Part model, mm, in its own coordinate system. A direction names the side the tool comes from. Round coordinates to 2 decimals unless told otherwise and drop trailing zeros. Write each loop counter-clockwise with the first axis right and the second up, starting at its lowest first coordinate (ties: lowest second). Pieces come first, ordered by that corner, then holes. Notation, with made-up numbers: M 73.25,75 L 132.25,75 A34 ccw 132.25,107 Z; hole C 9.5,-40 d10. An arc over 180 degrees is marked long. Answer as a JSON object with one key per item and string values. Group by question number.
1. Two-plate mould, pull along Y, no slides. Class faces 4 (the face through (19, -3.175, 0)), 5 (the face through (34.93, 98.29, 0.14)), 6 (the face through (0.69, 81.82, -3.1)): +Y half, -Y half, draft (parallel to the pull), parting line (faces both ways), or undercut.
2. Drill centre lines: line 1 (Y direction, x = 7.5, z = -1); line 2 (Y direction, x = 16.5, z = 0.25) (3 decimals); line 3 (X direction, y = 22, z = -0.25). Where is each one in solid material? Low to high. Write a range as from..to.
3. Which spindle directions (+Z, -Z, +X, -X, +Y, -Y) get a long thin tool onto all of the face, cutting with end or side? Do faces 1 (the face through (38, 88.9, 0)), 2 (the face through (22.22, 11.77, 0.14)), 3 (the face through (11.521, 42.193, -1.932)). Say none if no direction does.
4. Drop flat-ended pins along their axis: pin 1 (1.9 mm diameter, centred on x = 39, z = 1.5, fed in from -Y); pin 2 (2 mm diameter, centred on y = 101.5, z = -2, fed in from +X); pin 3 (1 mm diameter, centred on x = 23.5, y = 19.5, fed in from +Z). Give the stop position or say it passes through.
5. Band-saw the part on A-A, the plane z = 0. Write the cut outline in (x, y) (3 decimals).
6. Band-saw the part on B-B, the plane y = 75. Write the cut outline in (x, z) (3 decimals), plus the area to 3 significant figures.
Autodesk Inventor part; units mm, degrees
ref_plane "Work Plane1" through (19.05, 0, 0) normal (0, 1, 0) x (-1, 0, 0)
ref_plane "YZ Plane" through (0, 0, 0) normal (1, 0, 0) x (0, 1, 0)
ref_plane "XZ Plane" through (0, 0, 0) normal (0, 1, 0) x (-1, 0, 0)
sketch "Sketch1" plane through (0, 0, 0) normal (0, 0, 1) x (1, 0, 0)
  line L0 (19.05, 0) -> (19.05, 25.4)
  line L1 (19.05, 25.4) -> (0, 55.8663)
  arc A0 (38.1, 107.95) -> (0, 107.95) centre (19.05, 107.95) ccw
  line L2 (0, 55.8663) -> (0, 107.95)
  line L3 (38.1, 88.9) -> (38.1, 107.95)
  point P0 (0, 0)
  dimension "d2" = 25.4
ref_plane "Work Plane1" through (19.05, 0, 0) normal (0, 1, 0) x (-1, 0, 0)
sketch "Sketch2" plane through (19.05, 0, 0) normal (0, 1, 0) x (-1, 0, 0)
  circle A0 centre (0, 0) radius 3.175
  point P0 (19.05, 0)
  dimension "d6" = 6.35
sweep "Sweep1" add profiles "Sketch2" path "Sketch1"
sketch "Sketch3" plane through (19.05, 0, 0) normal (0, 1, 0) x (-1, 0, 0)
  circle A0 centre (0, 0) radius 3.175
  point P0 (19.05, 0)
  dimension "d8" = 6.35
extrude "Extrusion1" add sketch "Sketch3" against normal blind 3.175
ref_plane "Work Plane3" through (19.05, 11.1125, 0) normal (0, -1, 0) x (1, 0, 0)
ref_plane "Work Plane2" through (19.05, -3.175, 0) normal (0, -1, 0) x (1, 0, 0)
split_face "Split1"
thread "Thread1"
sketch "Sketch4" plane through (38.1, 88.9, 0) normal (0, -1, 0) x (1, 0, 0)
  circle A0 centre (0, 0) radius 3.175
  point P0 (-38.1, 0)
  point P1 (3.175, 0)
  point P2 (-3.1732, -0.1068)
sketch "Sketch5" plane through (19.05, -3.175, 0) normal (0, -1, 0) x (1, 0, 0)
  circle A0 centre (0, 0) radius 3.175
  point P0 (-19.05, 0)
  point P1 (3.175, 0)
ref_plane "Work Plane6" through (41.275, 88.9, 0) normal (-0.0168, 0.0035, 0.9999) x (-0.9999, 0, -0.0168)
properties part number "hook prototype"
Worked answers:
{
 "1": {"face 4": "-Y half", "face 5": "draft", "face 6": "undercut"},
 "2": {"line 1": "y = 38.19..49.56, 119.08..126.75", "line 2": "y = -3.175..35.448, 123.629..130.018", "line 3": "x = 15.88..22.22"},
 "3": {"face 1": "+Z, -Z, +X, -Y", "face 2": "-Y", "face 3": "none"},
 "4": {"pin 1": "stops at y = 88.9", "pin 2": "stops at x = 41.11", "pin 3": "passes through"},
 "5": {"outline": "M -3.175,54.955 L 15.875,24.489 L 15.875,-3.175 L 22.225,-3.175 L 22.225,26.311 L 3.175,56.777 L 3.175,107.95 A15.875 cw 34.925,107.95 L 34.925,88.9 L 41.275,88.9 L 41.275,107.95 A22.225 ccw -3.175,107.95 Z"},
 "6": {"outline": "C 0,0 d6.35", "area": "31.7 mm^2"}
}
